Work out the finished part from the listing and answer in its coordinate system (mm). A direction names the side the tool comes from. Round coordinates to 2 decimals unless told otherwise and drop trailing zeros. Write each loop counter-clockwise with the first axis right and the second up, starting at its lowest first coordinate (ties: lowest second). Pieces come first, ordered by that corner, then holes.
1. A tool of negligible diameter and unlimited length cuts with its end or side. For faces 1 (the face through (137, 6, 0)), 2 (the face through (0.5, 6, 12)), from which of +Z, -Z, +X, -X, +Y, -Y can it reach the whole face along a straight path? Write none if from no direction.
2. Find section B-B (x = 194). Write down the section's boundary in (y, z), and give its area (3 significant figures).
3. Flat-ended cylindrical pins translate along their axes: pin 1 Ø1 at (y, z) = (379.5, -0.5) entering from -X; pin 2 Ø1 at (y, z) = (-379.5, -1) entering from -X; pin 3 Ø1 at (y, z) = (119.5, 18) entering from +X. Find the tip coordinate at first contact, or state that the pin passes through.
4. Find section C-C (y = -350.5). Write down the section's boundary in (x, z), and give its area (3 significant figures).
5. Find section A-A (y = 129). Write down the section's boundary in (x, z).
6. Straight lines are drawn through the part: probe 1 along Z at (x, y) = (41, -350.5); probe 2 along X at (y, z) = (-270.5, 1); probe 3 along X at (y, z) = (364.5, -0.5). For each, find the intervals that lie inside material, in ascending order.
```python
from build123d import *

# Parameters (mm, degrees)
SKETCH_1_W                       = 550
SKETCH_1_H                       = 800
SM_BASE_FLANGE_1_DEPTH           = 2
SKETCH_6_W                       = 40
SKETCH_6_H                       = 130
CUT_EXTRUDE_1_DEPTH              = 10
FILLET_1_R                       = 5
SKETCH_7_W                       = 1
SKETCH_7_H                       = 845.505579408
CUT_EXTRUDE_2_DEPTH              = 10
SKETCH_8_W                       = 316.431651149
SKETCH_8_H                       = 807.863383274
CUT_EXTRUDE_3_DEPTH              = 10
SM_EDGE_FLANGE_1_STRIP_W         = 9.4732
SM_EDGE_FLANGE_1_STRIP_H         = 2
SM_EDGE_FLANGE_1_STRIP_CUT_DEPTH = 800
SM_EDGE_FLANGE_1_DEPTH           = 800
FILLET_2_R                       = 5
CUT_EXTRUDE_4_DEPTH              = 10
SKETCH_13_R                      = 3
CUT_EXTRUDE_5_DEPTH              = 10
PATTERN_LINEAR_1_COUNT           = 6
PATTERN_LINEAR_1_PITCH           = 150


# Sheet-metal steps are written as plain solids
with BuildPart() as part:
    # Sketch 1 → 基体-法兰1 (new body)
    with BuildSketch(Plane.XY):
        Rectangle(SKETCH_1_W, SKETCH_1_H)
    extrude(amount=-SM_BASE_FLANGE_1_DEPTH)

    # 草图6 → 切除-拉伸1 (cut)
    with BuildSketch(Plane.XY):
        with Locations((255, 335)):
            Rectangle(SKETCH_6_W, SKETCH_6_H)
        with Locations((255, -335)):
            Rectangle(SKETCH_6_W, SKETCH_6_H)
    extrude(amount=-CUT_EXTRUDE_1_DEPTH, mode=Mode.SUBTRACT)

    # 圆角1
    fillet_1_edges = [part.edges().sort_by_distance(p)[0] for p in [
        (275, 270, -1),
        (235, 270, -1),
        (235, 400, -1),
        (275, -270, -1),
        (235, -400, -1),
        (235, -270, -1),
        (-275, 400, -1),
        (-275, -400, -1),
    ]]
    fillet(fillet_1_edges, radius=FILLET_1_R)

    # 草图7 → 切除-拉伸2 (cut)
    with BuildSketch(Plane.XY):
        Rectangle(SKETCH_7_W, SKETCH_7_H)
    extrude(amount=-CUT_EXTRUDE_2_DEPTH, mode=Mode.SUBTRACT)


with BuildPart() as cut_extrude_2_piece_1:
    # of the separate pieces the step leaves, piece 1, a body of its own (cut_extrude_2_pieces)
    add(part.part.solids().sort_by_distance((-0.5, -400, 0))[0])

    # 草图8 → 切除-拉伸3 (cut)
    with BuildSketch(Plane.XY):
        with Locations((-158.715825575, -3.931691637)):
            Rectangle(SKETCH_8_W, SKETCH_8_H)
    extrude(amount=-CUT_EXTRUDE_3_DEPTH, mode=Mode.SUBTRACT)


with BuildPart() as cut_extrude_2_piece_2:
    # of the separate pieces the step leaves, piece 2, a body of its own (cut_extrude_2_pieces)
    add(part.part.solids().sort_by_distance((230, -400, 0))[0])

    # 边线-法兰1 strip (across the edge) → 边线-法兰1 strip cut (cut)
    with BuildSketch(Plane(origin=(0.5, 400, 0), x_dir=(1, 0, 0), z_dir=(0, -1, 0))):
        with Locations((-2, -1)):
            Rectangle(SM_EDGE_FLANGE_1_STRIP_W, SM_EDGE_FLANGE_1_STRIP_H)
    extrude(amount=SM_EDGE_FLANGE_1_STRIP_CUT_DEPTH, mode=Mode.SUBTRACT)

    # 边线-法兰1 section (across the edge) → 边线-法兰1 (add)
    with BuildSketch(Plane(origin=(0.5, 400, 0), x_dir=(1, 0, 0), z_dir=(0, -1, 0))):
        with BuildLine():
            Line((0, 0.7366), (0, 23))
            Line((0, 23), (2, 23))
            Line((2, 23), (2, 0.7366))
            ThreePointArc((2, 0.7366), (2.215745145, 0.215745145), (2.7366, 0))
            Line((2.7366, 0), (2.7366, -2))
            ThreePointArc((2.7366, -2), (0.801531583, -1.198468417), (0, 0.7366))
        make_face()
    extrude(amount=SM_EDGE_FLANGE_1_DEPTH)

    # 圆角2
    fillet_2_edges = [cut_extrude_2_piece_2.edges().sort_by_distance(p)[0] for p in [
        (1.5, 400, 23),
        (1.5, -400, 23),
    ]]
    fillet(fillet_2_edges, radius=FILLET_2_R)

    # 草图12 → 切除-拉伸4 (cut)
    with BuildSketch(Plane.XY):
        with BuildLine():
            Line((51.5, 375), (51.5, 385))
            ThreePointArc((51.5, 385), (55, 388.5), (58.5, 385))
            Line((58.5, 385), (58.5, 375))
            ThreePointArc((58.5, 375), (55, 371.5), (51.5, 375))
        make_face()
        with BuildLine():
            Line((171.5, 375), (171.5, 385))
            ThreePointArc((171.5, 385), (175, 388.5), (178.5, 385))
            Line((178.5, 385), (178.5, 375))
            ThreePointArc((178.5, 375), (175, 371.5), (171.5, 375))
        make_face()
        with BuildLine():
            Line((51.5, -385), (51.5, -375))
            ThreePointArc((51.5, -375), (55, -371.5), (58.5, -375))
            Line((58.5, -375), (58.5, -385))
            ThreePointArc((58.5, -385), (55, -388.5), (51.5, -385))
        make_face()
        with BuildLine():
            Line((171.5, -385), (171.5, -375))
            ThreePointArc((171.5, -375), (175, -371.5), (178.5, -375))
            Line((178.5, -375), (178.5, -385))
            ThreePointArc((178.5, -385), (175, -388.5), (171.5, -385))
        make_face()
    extrude(amount=-CUT_EXTRUDE_4_DEPTH, mode=Mode.SUBTRACT)

    # 草图13 → 切除-拉伸5 (cut)
    with BuildSketch(Plane(origin=(2.5, 0, 0), x_dir=(0, 0, -1), z_dir=(1, 0, 0))):
        with Locations((-11, -375)):
            Circle(SKETCH_13_R)
    cut_extrude_5 = extrude(amount=-CUT_EXTRUDE_5_DEPTH, mode=Mode.SUBTRACT)

    # 阵列(线性)1: 切除-拉伸5 ×6
    with Locations(*[(0, i * PATTERN_LINEAR_1_PITCH, 0) for i in range(1, PATTERN_LINEAR_1_COUNT)]):
        add(cut_extrude_5, mode=Mode.SUBTRACT)


solid = cut_extrude_2_piece_2.part
```
Worked answers:
1. face 1: +Z, +X, +Y, -Y
1. face 2: +Z, -Z, -X, +Y, -Y
2. outline: (-400, -2) - (400, -2) - (400, 0) - (-400, 0) - close
2. area: 1,600 mm2
3. pin 1: stops at x = 0.6
3. pin 2: stops at x = 0.8
3. pin 3: stops at x = 2.5
4. outline: (0.5, 0.74) arc R2.74 ccw to (3.24, -2) - (235, -2) - (235, 0) - (3.24, 0) arc R0.74 cw to (2.5, 0.74) - (2.5, 23) - (0.5, 23) - close
4. area: 514 mm2
5. outline: (0.5, 0.74) arc R2.74 ccw to (3.24, -2) - (275, -2) - (275, 0) - (3.24, 0) arc R0.74 cw to (2.5, 0.74) - (2.5, 23) - (0.5, 23) - close
6. probe 1: z = -2 to 0
6. probe 2: x = 0.5 to 2.5
6. probe 3: x = 0.8 to 235
